Verification items for the finished model (mm, model axes). Round coordinates to 2 decimals unless told otherwise and drop trailing zeros. Write each loop counter-clockwise with the first axis right and the second up, starting at its lowest first coordinate (ties: lowest second). Pieces come first, ordered by that corner, then holes. Notation, with made-up numbers: M 85.5,36 L 107.5,36 A24 ccw 107.5,65 Z; hole C 53,75 d5. An arc over 180 degrees is marked long. One line per item, written item: value. Start each with the question number.
Item 1: Section check B-B, the plane x = 10. Record the cut outline in (y, z).
Item 2: Thickness scan on probe 1 along Y at (x, z) = (2.5, 4); probe 2 along Y at (x, z) = (10, 2.2); probe 3 along X at (y, z) = (47, 4.7). Record the ranges inside material, lowest first. Write a range as from..to.
Item 3: Section check C-C, the plane x = 2.5. Record the cut outline in (y, z).
Item 4: Section check A-A, the plane y = 12. Record the cut outline in (x, z).
Item 5: Gauge pin test, flat end, axial feed: pin 1 (1.5 mm diameter, centred on y = 7.5, z = 2.5, fed in from +X). Record the tip position at first contact, or that the pin passes through.
Item 6: Section check D-D, the plane z = 2.75. State how many separate pieces and enclosed holes the cut face has, then the cut area to 3 significant figures.
from build123d import *

# Parameters (mm, degrees)
SKETCH1_W           = 24
SKETCH1_H           = 110
SKETCH1_R           = 1.5
BOSS_EXTRUDE1_DEPTH = 5
SKETCH2_W           = 6
SKETCH2_H           = 37
SKETCH2_H_2         = 17
CUT_EXTRUDE1_DEPTH  = 113.698713391
BOSS_EXTRUDE2_DEPTH = 5
SKETCH4_R           = 1.5
SKETCH4_W           = 5
SKETCH4_H           = 10
CUT_EXTRUDE2_DEPTH  = 115.651646303
FILLET1_R           = 2
FILLET2_R           = 8
SKETCH5_W           = 7.5
SKETCH5_H           = 5.5
CUT_EXTRUDE3_DEPTH  = 115.651646303


with BuildPart() as part:
    # Sketch1 → Boss-Extrude1 (new body)
    with BuildSketch(Plane.XY):
        with Locations((12, 55)):
            Rectangle(SKETCH1_W, SKETCH1_H)
        with Locations((10, 12)):
            Circle(SKETCH1_R, mode=Mode.SUBTRACT)
        with Locations((10, 95)):
            Circle(SKETCH1_R, mode=Mode.SUBTRACT)
        with BuildLine():
            Line((4, 103.5), (4, 106.5))
            ThreePointArc((4, 106.5), (5.25, 107.75), (6.5, 106.5))
            Line((6.5, 106.5), (6.5, 103.5))
            ThreePointArc((6.5, 103.5), (5.25, 102.25), (4, 103.5))
        make_face(mode=Mode.SUBTRACT)
        with BuildLine():
            Line((11.5, 103.5), (11.5, 106.5))
            ThreePointArc((11.5, 106.5), (12.75, 107.75), (14, 106.5))
            Line((14, 106.5), (14, 103.5))
            ThreePointArc((14, 103.5), (12.75, 102.25), (11.5, 103.5))
        make_face(mode=Mode.SUBTRACT)
    extrude(amount=BOSS_EXTRUDE1_DEPTH)

    # Sketch2 → Cut-Extrude1 (cut, through all)
    with BuildSketch(Plane.XY.offset(5)):
        with Locations((21, 91.5)):
            Rectangle(SKETCH2_W, SKETCH2_H)
        with Locations((21, 8.5)):
            Rectangle(SKETCH2_W, SKETCH2_H_2)
    extrude(amount=-CUT_EXTRUDE1_DEPTH, mode=Mode.SUBTRACT)

    # Sketch3 → Boss-Extrude2 (add)
    with BuildSketch(Plane.XY.offset(5)):
        Polygon((18, -2), (18, 0), (0, 0), (0, 110), (18, 110), (18, 112), (-2, 112), (-2, -2), align=None)
    extrude(amount=-BOSS_EXTRUDE2_DEPTH)

    # Sketch4 → Cut-Extrude2 (cut, through all)
    with BuildSketch(Plane.XY.offset(5)):
        with Locations((2.5, 20)):
            Circle(SKETCH4_R)
        with Locations((2.5, 70)):
            Circle(SKETCH4_R)
        with Locations((2.5, 5)):
            Rectangle(SKETCH4_W, SKETCH4_H)
        with Locations((2.5, 85)):
            Rectangle(SKETCH4_W, SKETCH4_H)
        with Locations((2.5, 45)):
            Rectangle(SKETCH4_W, SKETCH4_H)
    extrude(amount=-CUT_EXTRUDE2_DEPTH, mode=Mode.SUBTRACT)

    # Fillet1
    fillet1_edges = [part.edges().sort_by_distance(p)[0] for p in [
        (18, 112, 2.5),
        (-2, 112, 2.5),
        (-2, -2, 2.5),
        (18, -2, 2.5),
    ]]
    fillet(fillet1_edges, radius=FILLET1_R)

    # Fillet2
    # the kernel refuses this fillet: 8 mm, written as the material it takes off along each edge
    with BuildSketch(Plane(origin=(24, 17, 24.364916731), x_dir=(0, 1, 0), z_dir=(0, 0, -1))) as fillet2_piece_1:
        with BuildLine():
            CenterArc((7.745966692, -8), FILLET2_R, 90, 75.522487814)
            Line((0, -6), (-0.154919334, -5.96))
            ThreePointArc((-0.154919334, -5.96), (-0.16, -3), (-0.16, 0))
            Line((-0.16, 0), (0, 0.16))
            Line((0, 0.16), (7.745966692, 0.16))
            Line((7.745966692, 0.16), (7.745966692, 0))
        make_face()
    extrude(amount=43.729833462, mode=Mode.SUBTRACT)
    with BuildSketch(Plane(origin=(24, 73, 24.364916731), x_dir=(-1, 0, 0), z_dir=(0, 0, -1))) as fillet2_piece_2:
        with BuildLine():
            CenterArc((8, -7.745966692), FILLET2_R, 104.477512186, 75.522487814)
            Line((0, -7.745966692), (-0.16, -7.745966692))
            Line((-0.16, -7.745966692), (-0.16, 0))
            Line((-0.16, 0), (0, 0.16))
            ThreePointArc((0, 0.16), (3, 0.16), (5.96, 0.154919334))
            Line((5.96, 0.154919334), (6, 0))
        make_face()
    extrude(amount=43.729833462, mode=Mode.SUBTRACT)

    # Sketch5 → Cut-Extrude3 (cut, through all)
    with BuildSketch(Plane.XY.offset(5)):
        with Locations((9, 105)):
            Rectangle(SKETCH5_W, SKETCH5_H)
    extrude(amount=-CUT_EXTRUDE3_DEPTH, mode=Mode.SUBTRACT)


solid = part.part
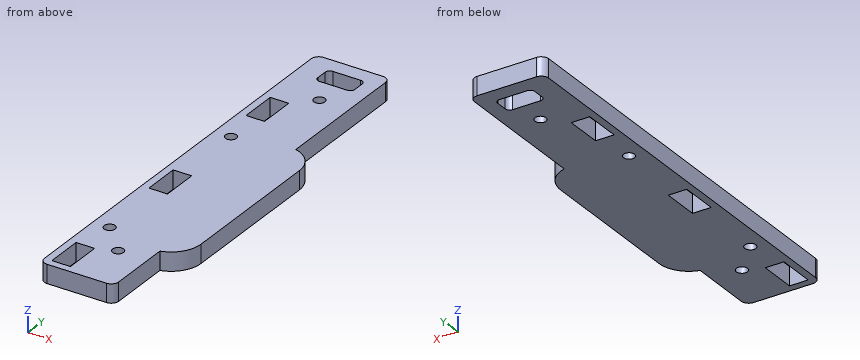
Response values:
1. outline: M -2,0 L 10.5,0 L 10.5,5 L -2,5 Z; M 13.5,0 L 93.5,0 L 93.5,5 L 13.5,5 Z; M 96.5,0 L 102.25,0 L 102.25,5 L 96.5,5 Z; M 107.75,0 L 112,0 L 112,5 L 107.75,5 Z
2. probe 1: y = -2..0, 10..18.5, 21.5..40, 50..68.5, 71.5..80, 90..112
2. probe 2: y = -2..10.5, 13.5..93.5, 96.5..102.25, 107.75..112
2. probe 3: x = -2..0, 5..24
3. outline: M -2,0 L 0,0 L 0,5 L -2,5 Z; M 10,0 L 18.5,0 L 18.5,5 L 10,5 Z; M 21.5,0 L 40,0 L 40,5 L 21.5,5 Z; M 50,0 L 68.5,0 L 68.5,5 L 50,5 Z; M 71.5,0 L 80,0 L 80,5 L 71.5,5 Z; M 90,0 L 112,0 L 112,5 L 90,5 Z
4. outline: M -2,0 L 8.5,0 L 8.5,5 L -2,5 Z; M 11.5,0 L 18,0 L 18,5 L 11.5,5 Z
5. pin 1: stops at x = 18
6. separate pieces: 1
6. enclosed holes: 8
6. area: 2,360 mm2
